from build123d import *

# Parameters (mm, degrees)
ESKIZ_KONTUR_W        = 12.6
ESKIZ_KONTUR_H        = 23.2
PLASTINA_DEPTH        = 3
OTVERSTIYA_DEPTH      = 33.664965942
OTVERSTIYA_DEPTH_BACK = 33.664965942
ESKIZ_OTVERSTIYA_R    = 1.1


with BuildPart() as part:
    # Eskiz_kontur → Plastina (new body)
    with BuildSketch(Plane.XY):
        Polygon((20, -3.35), (15.5, -3.35), (15.5, -2.1), (12.9, -2.1), (12.9, -3.35), (10, -3.35), (10, -6.65), (12.9, -6.65), (12.9, -7.9), (15.5, -7.9), (15.5, -6.65), (20, -6.65), (20, -12), (23, -12), (23, -20), (20, -20), (20, -23), (-20, -23), (-20, -20), (-23, -20), (-23, -12), (-20, -12), (-20, -6.65), (-15.5, -6.65), (-15.5, -7.9), (-12.9, -7.9), (-12.9, -6.65), (-10, -6.65), (-10, -3.35), (-12.9, -3.35), (-12.9, -2.1), (-15.5, -2.1), (-15.5, -3.35), (-20, -3.35), (-20, 2), (-23, 2), (-23, 10), (-20, 10), (-20, 12), (20, 12), (20, 10), (23, 10), (23, 2), (20, 2), align=None)
        with Locations((0, -5.4)):
            Rectangle(ESKIZ_KONTUR_W, ESKIZ_KONTUR_H, mode=Mode.SUBTRACT)
    extrude(amount=PLASTINA_DEPTH)

    # Eskiz_otverstiya → Otverstiya (cut, two sides: drawn at the far end of the back side and taken through both)
    with BuildSketch(Plane.XY.offset(-OTVERSTIYA_DEPTH_BACK)):
        with Locations((0, -19.3)):
            Circle(ESKIZ_OTVERSTIYA_R)
        with Locations((0, 8.5)):
            Circle(ESKIZ_OTVERSTIYA_R)
    extrude(amount=OTVERSTIYA_DEPTH + OTVERSTIYA_DEPTH_BACK, mode=Mode.SUBTRACT)


solid = part.part
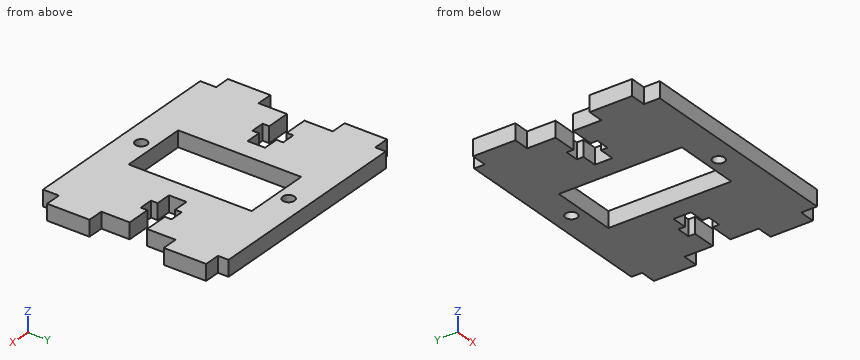
Input: part model. Units: mm. Frame: model coordinates. Coordinates: 2 decimals unless noted, no trailing zeros. Loops run counter-clockwise (first coordinate to the right, second up) from the corner with the lowest first, then second, coordinate; pieces in that order, holes last.
Q1. Material intervals for line 1 (Y direction, x = 0, z = 1.65); line 2 (Y direction, x = -14.5, z = 1.7); line 3 (Y direction, x = 6, z = 2), sorted ascending.
Q2. Contact query for a flat-ended pin moving along its axis: pin 1 (1.6 mm diameter, centred on y = 11.5, z = 1.5, fed in from -X). Output: stop coordinate, or through.
Q3. Cut plane D-D (z = 2.2). Give the number of separate pieces and of enclosed holes in the cut face, then the cut area to 3 significant figures.
Q4. Cut plane B-B (x = -18). Output: boundary loops of the cut face in (y, z).
Q5. Cut plane C-C (x = 0). Output: boundary loops of the cut face in (y, z), then the cut area to 3 significant figures.
Q6. Cut plane A-A (y = 8.5). Output: boundary loops of the cut face in (x, z).
Working result:
1. line 1: y = -23 to -20.4, -18.2 to -17, 6.2 to 7.4, 9.6 to 12
1. line 2: y = -23 to -7.9, -2.1 to 12
1. line 3: y = -23 to -17, 6.2 to 12
2. pin 1: stops at x = -20
3. separate pieces: 1
3. enclosed holes: 3
3. area: 1,120 mm2
4. outline: (-23, 0) - (-6.65, 0) - (-6.65, 3) - (-23, 3) - close; (-3.35, 0) - (12, 0) - (12, 3) - (-3.35, 3) - close
5. outline: (-23, 0) - (-20.4, 0) - (-20.4, 3) - (-23, 3) - close; (-18.2, 0) - (-17, 0) - (-17, 3) - (-18.2, 3) - close; (6.2, 0) - (7.4, 0) - (7.4, 3) - (6.2, 3) - close; (9.6, 0) - (12, 0) - (12, 3) - (9.6, 3) - close
5. area: 22.2 mm2
6. outline: (-23, 0) - (-1.1, 0) - (-1.1, 3) - (-23, 3) - close; (1.1, 0) - (23, 0) - (23, 3) - (1.1, 3) - close
